Autodesk Inventor part; units mm, degrees
ref_plane "YZ Plane" through (0, 0, 0) normal (1, 0, 0) x (0, 1, 0)
ref_plane "XZ Plane" through (0, 0, 0) normal (0, 1, 0) x (-1, 0, 0)
ref_plane "XY Plane" through (0, 0, 0) normal (0, 0, 1) x (1, 0, 0)
sketch "Sketch1" plane through (0, 0, 0) normal (0, 1, 0) x (-1, 0, 0)
  line L0 (0, 0) -> (152.4, 0)
  line L1 (152.4, 0) -> (152.4, -31.75)
  line L2 (152.4, -31.75) -> (0, -31.75)
  line L3 (0, -31.75) -> (0, 0)
  line L4 (127, -8.89) -> (96.52, -8.89)
  line L5 (96.52, -8.89) -> (96.52, -22.86)
  line L6 (96.52, -22.86) -> (127, -22.86)
  line L7 (127, -22.86) -> (127, -8.89)
  line L8 (117.2368, -8.89) -> (117.2368, 0)
  line L9 (117.2368, -22.86) -> (117.2368, -31.75)
  dimension "d0" = 152.4
  dimension "d1" = 31.75
  dimension "d2" = 30.48
  dimension "d3" = 13.97
  dimension "d4" = 25.4
extrude "Extrusion1" add sketch "Sketch1" along normal blind 1.778 contours L0 L8 L4 L5 L6 L9 L2 L3 | L0 L1 L2 L9 L6 L7 L4 L8
sketch "Sketch2" plane through (0, 0, 0) normal (0, -1, 0) x (1, 0, 0)
  line L0 (-152.4, 0) -> (0, 0)
  line L1 (0, 0) -> (0, -31.75)
  line L2 (-152.4, 0) -> (0, 0)
  line L3 (0, 0) -> (0, -31.75)
  line L4 (0, -31.75) -> (-152.4, -31.75)
  line L5 (-152.4, -31.75) -> (-152.4, 0)
  line L6 (-127, -2.7348) -> (-96.52, -2.7348)
  line L7 (-96.52, -2.7348) -> (-96.52, -29.0152)
  line L8 (-96.52, -29.0152) -> (-127, -29.0152)
  line L9 (-127, -29.0152) -> (-127, -2.7348)
  line L10 (-127, -8.89) -> (-127, -22.86)
  line L11 (-103.8171, -2.7348) -> (-103.8171, 0)
  line L12 (-104.7941, -29.0152) -> (-104.7941, -31.75)
  line L13 (0, -31.75) -> (-152.4, -31.75)
  dimension "d7" = 30.48
  dimension "d8" = 0
extrude "Extrusion2" add sketch "Sketch2" along normal blind 1.778 contours L0 L11 L6 L9 L8 L12 L4 L5 | L0 L1 L4 L12 L8 L7 L6 L11
sketch "Sketch3" plane through (0, -1.778, 0) normal (0, -1, 0) x (1, 0, 0)
  line L0 (-152.4, 0) -> (0, 0)
  line L1 (0, -31.75) -> (-152.4, -31.75)
  line L2 (-152.4, 0) -> (0, 0)
  line L3 (0, 0) -> (0, -31.75)
  line L4 (0, -31.75) -> (-152.4, -31.75)
  line L5 (-152.4, -31.75) -> (-152.4, 0)
  line L6 (-1.5875, -30.1625) -> (-1.5875, -1.5875)
  line L7 (-1.5875, -1.5875) -> (-150.8125, -1.5875)
  line L8 (-150.8125, -1.5875) -> (-150.8125, -30.1625)
  line L9 (-150.8125, -30.1625) -> (-1.5875, -30.1625)
  dimension "d11" = 1.5875
extrude "Extrusion3" add sketch "Sketch3" along normal blind 6.35
sketch "Sketch4" plane through (0, 1.778, 0) normal (0, 1, 0) x (1, 0, 0)
  line L0 (-152.4, 0) -> (0, 0)
  line L1 (-152.4, 31.75) -> (-152.4, 0)
  line L2 (0, 0) -> (-152.4, 0)
  line L3 (-152.4, 0) -> (-152.4, 31.75)
  line L4 (-152.4, 31.75) -> (0, 31.75)
  line L5 (-6.35, 25.4) -> (-146.05, 25.4)
  line L6 (-146.05, 25.4) -> (-146.05, 6.35)
  line L7 (-146.05, 6.35) -> (-6.35, 6.35)
  line L8 (-13.5859, 25.4) -> (0, 25.4)
  line L9 (0, 0) -> (0, 31.75)
  line L10 (-13.5859, 6.35) -> (0, 6.35)
  line L11 (0, 31.75) -> (0, 25.4)
  line L12 (0, 6.35) -> (0, 0)
  line L13 (-127, 22.86) -> (-96.52, 22.86)
  line L14 (-96.52, 22.86) -> (-93.98, 22.86)
  line L15 (-93.98, 22.86) -> (-93.98, 25.4)
  line L16 (-93.98, 25.4) -> (-96.52, 25.4)
  line L17 (-96.52, 25.4) -> (-96.52, 22.86)
  line L18 (-96.52, 2.7348) -> (-96.52, 29.0152)
  line L19 (-96.52, 6.35) -> (-93.98, 6.35)
  line L20 (-93.98, 6.35) -> (-93.98, 8.89)
  line L21 (-93.98, 8.89) -> (-96.52, 8.89)
  line L22 (-96.52, 8.89) -> (-96.52, 6.35)
  line L23 (-121.92, 25.4) -> (-124.46, 25.4)
  line L24 (-124.46, 25.4) -> (-124.46, 22.86)
  line L25 (-124.46, 22.86) -> (-121.92, 22.86)
  line L26 (-121.92, 22.86) -> (-121.92, 25.4)
  line L27 (-121.92, 6.35) -> (-124.46, 6.35)
  line L28 (-124.46, 6.35) -> (-124.46, 8.89)
  line L29 (-124.46, 8.89) -> (-121.92, 8.89)
  line L30 (-121.92, 8.89) -> (-121.92, 6.35)
  line L31 (-68.58, 25.4) -> (-66.04, 25.4)
  line L32 (-66.04, 25.4) -> (-66.04, 22.86)
  line L33 (-66.04, 22.86) -> (-68.58, 22.86)
  line L34 (-68.58, 22.86) -> (-68.58, 25.4)
  line L35 (-68.58, 6.35) -> (-66.04, 6.35)
  line L36 (-66.04, 6.35) -> (-66.04, 8.89)
  line L37 (-66.04, 8.89) -> (-68.58, 8.89)
  line L38 (-68.58, 8.89) -> (-68.58, 6.35)
  line L39 (-40.64, 6.35) -> (-38.1, 6.35)
  line L40 (-38.1, 6.35) -> (-38.1, 8.89)
  line L41 (-38.1, 8.89) -> (-40.64, 8.89)
  line L42 (-40.64, 8.89) -> (-40.64, 6.35)
  line L43 (-40.64, 25.4) -> (-38.1, 25.4)
  line L44 (-38.1, 25.4) -> (-38.1, 22.86)
  line L45 (-38.1, 22.86) -> (-40.64, 22.86)
  line L46 (-40.64, 22.86) -> (-40.64, 25.4)
  line L47 (-12.7, 25.4) -> (-10.16, 25.4)
  line L48 (-10.16, 25.4) -> (-10.16, 22.86)
  line L49 (-10.16, 22.86) -> (-12.7, 22.86)
  line L50 (-12.7, 22.86) -> (-12.7, 25.4)
  line L51 (-12.7, 6.35) -> (-10.16, 6.35)
  line L52 (-10.16, 6.35) -> (-10.16, 8.89)
  line L53 (-10.16, 8.89) -> (-12.7, 8.89)
  line L54 (-12.7, 8.89) -> (-12.7, 6.35)
  point P0 (-121.92, 7.62)
  point P1 (-96.52, 7.62)
  point P2 (-93.98, 24.13)
  point P3 (-68.58, 24.13)
  point P4 (-40.64, 24.13)
  point P5 (-66.04, 24.13)
  point P6 (-12.7, 24.13)
  point P7 (-38.1, 24.13)
  point P8 (-6.35, 6.35)
  dimension "d14" = 6.35
  dimension "d15" = 2.54
  dimension "d16" = 2.54
  dimension "d17" = 2.54
  dimension "d18" = 2.54
  dimension "d19" = 2.54
  dimension "d20" = 2.54
  dimension "d21" = 25.4
  dimension "d22" = 2.54
  dimension "d23" = 2.54
  dimension "d24" = 2.54
  dimension "d25" = 2.54
  dimension "d26" = 2.54
  dimension "d27" = 2.54
  dimension "d28" = 2.54
  dimension "d29" = 2.54
  dimension "d30" = 2.54
  dimension "d31" = 2.54
  dimension "d32" = 2.54
  dimension "d33" = 2.54
  dimension "d34" = 25.4
  dimension "d35" = 25.4
  dimension "d36" = 25.4
extrude "Extrusion4" add sketch "Sketch4" along normal blind 31.75 contours L1 L4 L9 L8 L5 L6 L7 L10 L0 | L7 L54 L53 L52 | L48 L49 L50 L5 | L7 L42 L41 L40 | L44 L45 L46 L5 | L7 L38 L37 L36 | L32 L33 L34 L5 | L7 L18 L21 L20 | L15 L14 L17 L5 | L7 L28 L29 L30 | L26 L13 L24 L5
sketch "Sketch5" plane through (-93.98, 1.778, -8.89) normal (0, 0, -1) x (-1, 0, 0)
  line L0 (2.54, 31.75) -> (0, 31.75)
  line L1 (0, 31.75) -> (0, 29.21)
  line L2 (0, 29.21) -> (2.54, 29.21)
  line L3 (2.54, 29.21) -> (2.54, 31.75)
  line L4 (30.48, 31.75) -> (27.94, 31.75)
  line L5 (30.48, 0) -> (30.48, 31.75)
  line L6 (27.94, 31.75) -> (30.48, 31.75)
  line L7 (30.48, 31.75) -> (30.48, 29.21)
  line L8 (30.48, 29.21) -> (27.94, 29.21)
  line L9 (27.94, 29.21) -> (27.94, 31.75)
  line L10 (-27.94, 0) -> (-27.94, 31.75)
  line L11 (-25.4, 0) -> (-25.4, 31.75)
  line L12 (-27.94, 29.21) -> (-25.4, 29.21)
  line L13 (-25.4, 29.21) -> (-25.4, 31.75)
  line L14 (-25.4, 31.75) -> (-27.94, 31.75)
  line L15 (-27.94, 31.75) -> (-27.94, 29.21)
  line L16 (-93.98, 31.75) -> (58.42, 31.75)
  line L17 (-27.94, 31.75) -> (-25.4, 31.75)
  line L18 (-25.4, 31.75) -> (-25.4, 29.21)
  line L19 (-25.4, 29.21) -> (-27.94, 29.21)
  line L20 (-27.94, 29.21) -> (-27.94, 31.75)
  line L21 (-53.34, 31.75) -> (-55.88, 31.75)
  line L22 (-55.88, 31.75) -> (-55.88, 29.21)
  line L23 (-55.88, 29.21) -> (-53.34, 29.21)
  line L24 (-53.34, 29.21) -> (-53.34, 31.75)
  line L25 (-81.28, 31.75) -> (-83.82, 31.75)
  line L26 (-83.82, 31.75) -> (-83.82, 29.21)
  line L27 (-83.82, 29.21) -> (-81.28, 29.21)
  line L28 (-81.28, 29.21) -> (-81.28, 31.75)
  line L29 (30.48, 31.75) -> (52.07, 31.75)
  line L30 (30.48, 31.75) -> (27.94, 31.75)
  line L31 (27.94, 31.75) -> (27.94, 29.21)
  line L32 (27.94, 29.21) -> (30.48, 29.21)
  line L33 (30.48, 29.21) -> (30.48, 31.75)
  point P0 (-93.98, -1.778)
  point P1 (0, 30.48)
  point P2 (-25.4, 30.48)
  point P3 (-27.94, 30.48)
  point P4 (-53.34, 30.48)
  point P5 (-81.28, 30.48)
  point P6 (-55.88, 30.48)
  point P7 (27.94, 30.48)
  point P8 (2.54, 30.48)
  dimension "d39" = 2.54
  dimension "d40" = 2.54
  dimension "d41" = 2.54
  dimension "d42" = 2.54
  dimension "d43" = 2.54
  dimension "d44" = 2.54
  dimension "d45" = 25.4
  dimension "d46" = 25.4
  dimension "d47" = 2.54
  dimension "d48" = 2.54
  dimension "d49" = 25.4
  dimension "d50" = 2.54
  dimension "d51" = 2.54
  dimension "d52" = 25.4
extrude "Extrusion5" add sketch "Sketch5" along normal up to next
sketch "Sketch6" plane through (0, 33.528, 0) normal (0, 1, 0) x (1, 0, 0)
  line L0 (-152.4, 31.75) -> (-152.4, 0)
  line L1 (0, 31.75) -> (-152.4, 31.75)
  line L2 (-152.4, 0) -> (0, 0)
  line L3 (0, 0) -> (0, 31.75)
  line L4 (0, 31.75) -> (-152.4, 31.75)
  line L5 (-152.4, 31.75) -> (-152.4, 0)
extrude "Extrusion6" add sketch "Sketch6" along normal blind 3.175
ref_plane "Work Plane1" through (-127, 1.778, -8.89) normal (0.7071, -0.7071, 0) x (0, 0, -1)
sketch "Sketch7" plane through (-127, 1.778, -8.89) normal (0.7071, -0.7071, 0) x (0, 0, -1)
  line L0 (20.1252, -1.2572) -> (20.1252, 20.2954)
  line L1 (20.1252, 0) -> (-6.1552, 0)
  line L2 (-6.1552, 0) -> (-6.1552, 127)
  line L3 (-6.1552, 127) -> (20.1252, 127)
  line L4 (20.1252, 127) -> (20.1252, 0)
  line L5 (0, 0) -> (13.97, 0)
  point P0 (-8.89, 88.5453)
  point P1 (20.1252, 20.2954)
  dimension "d58" = 0
  dimension "d59" = 127
extrude "Extrusion7" cut sketch "Sketch7" against normal blind 3.175
sketch "Sketch8" plane through (0, 1.778, 0) normal (0, 1, 0) x (1, 0, 0)
  line L0 (63.8737, 171.7375) -> (-193.0507, 171.7375)
  line L1 (-193.0507, 171.7375) -> (-193.0507, -76.4775)
  line L2 (-193.0507, -76.4775) -> (63.8737, -76.4775)
  line L3 (63.8737, -76.4775) -> (63.8737, 171.7375)
  point P0 (0, 0)
extrude "Extrusion8" cut sketch "Sketch8" against normal through all
properties part number "Top"
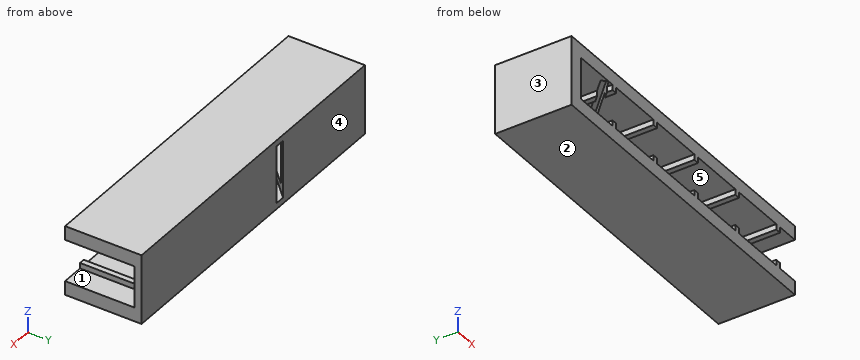
Geometry: final body of the model. Coordinates: model frame, mm. Face numbers are marked on the shaded views. A direction names the side the tool comes from. Coordinates: 2 decimals unless noted, no trailing zeros. Loops run counter-clockwise (first coordinate to the right, second up) from the corner with the lowest first, then second, coordinate; pieces in that order, holes last. Notation, with made-up numbers: M 50,-11 L 83,-11 A19 ccw 83,26 Z; hole C -10.75,-23 d4. An arc over 180 degrees is marked long. One line per item, written item: value. Start each with the question number.
1) Pin query (flat end, axial travel): P1, Ø2, axis at x = -39.5, z = -14, coming from the -Y side; P2, Ø2, axis at y = 17.5, z = -21, coming from the +X side; P3, Ø5.5, axis at x = -86, z = -12.5, coming from the -Y side. Return the tip coordinate at first contact, or that it passes through.
2) Material intervals for L1, parallel to X at y = 13.5, z = -6.5; L2, parallel to Z at x = -118.5, y = 7.5; L3, parallel to Z at x = -124, y = 12, sorted ascending. Write a range as from..to.
3) Cut plane C-C (x = -120). Return loops of the section in (y, z).
4) Draft query along Z for the marked faces 1, 2 and 3. Return one class per face: released by +Z, released by -Z, zero draft, split by the parting line, or undercut.
5) Cut plane B-B (x = -15). Return loops of the section in (y, z).
6) Reachability of the marked faces 4 and 5 from +Z, -Z, +X, -X, +Y, -Y: full face, straight path, thin tool, end or side. Return the list, or none.
Evaluation:
1. P1: y = 30.99
1. P2: x = -146.05
1. P3: y = 33.53
2. L1: -152.4..-146.05, -124.46..-121.92, -96.52..-93.98, -68.58..-66.04, -40.64..-38.1, -12.7..-10.16
2. L2: -31.75..-25.4, -6.35..0
2. L3: -31.75..-22.86, -8.89..0
3. outline: M 1.78,-31.75 L 36.7,-31.75 L 36.7,0 L 1.78,0 L 1.78,-6.35 L 8.78,-6.35 L 8.78,-2.73 L 13.27,-2.73 L 13.27,-6.35 L 33.53,-6.35 L 33.53,-25.4 L 13.27,-25.4 L 13.27,-29.02 L 8.78,-29.02 L 8.78,-25.4 L 1.78,-25.4 Z
4. face 1: undercut
4. face 2: released by -Z
4. face 3: zero draft
5. outline: M 1.78,-31.75 L 36.7,-31.75 L 36.7,0 L 1.78,0 L 1.78,-6.35 L 33.53,-6.35 L 33.53,-25.4 L 1.78,-25.4 Z
6. face 4: +Z, -Z, +X, -X, +Y
6. face 5: -Y
